Can you work these out from the model? Positions are in its coordinate system, mm. Coordinates: 2 decimals unless noted, no trailing zeros. Write each loop counter-clockwise with the first axis right and the second up, starting at its lowest first coordinate (ties: lowest second). Pieces come first, ordered by that corner, then holes.
```python
from build123d import *

# Parameters (mm, degrees)
SKETCH_1_W      = 200
SKETCH_1_H      = 5
EXTRUDE_1_DEPTH = 3


with BuildPart() as part:
    # 草图1 → 凸台-拉伸1 (new body)
    with BuildSketch(Plane.XY):
        Polygon((0, -80), (0, -100), (100, -100), (100, 0), (80, 0), (80, -3), (40, -3), (40, 0), (0, 0), (0, -40), (3, -40), (3, -80), align=None)
        Polygon((100, -100), (0, -100), (0, -120), (3, -120), (3, -160), (0, -160), (0, -200), (40, -200), (40, -197), (80, -197), (80, -200), (100, -200), align=None)
        Polygon((100, 0), (100, -100), (200, -100), (200, -80), (197, -80), (197, -40), (200, -40), (200, 0), (160, 0), (160, -3), (120, -3), (120, 0), align=None)
        Polygon((200, -100), (100, -100), (100, -200), (120, -200), (120, -197), (160, -197), (160, -200), (200, -200), (200, -160), (197, -160), (197, -120), (200, -120), align=None)
        Polygon((-5, -205), (-5, 5), (0, 5), (0, 0), (0, -200), (0, -205), align=None)
        with Locations((100, 2.5)):
            Rectangle(SKETCH_1_W, SKETCH_1_H)
        Polygon((205, 5), (205, -200), (200, -200), (200, 0), (200, 5), align=None)
        Polygon((0, -200), (200, -200), (205, -200), (205, -205), (0, -205), align=None)
    extrude(amount=EXTRUDE_1_DEPTH)


solid = part.part
```
1. If we section it at B-B, the plane x = 133.5: List the corners of the cut face in (y, z) for me.
2. If I drill on L1, parallel to X at y = -73.5, z = 1.2; L2, parallel to Y at x = 70, z = 0.55, over which ranges is the centre line in solid material (lowest first)?
3. If we section it at C-C, the plane z = 0.65: Count the separate pieces of the cut face and the enclosed holes in it, plus the area to 3 significant figures.
4. If we section it at A-A, the plane y = -75.5: List the corners of the cut face in (x, z) for me, plus the area to 3 significant figures.
Answers:
1. outline: (-205, 0) - (-200, 0) - (-200, 3) - (-205, 3) - close; (-197, 0) - (-3, 0) - (-3, 3) - (-197, 3) - close; (0, 0) - (5, 0) - (5, 3) - (0, 3) - close
2. L1: x = -5 to 0, 3 to 197, 200 to 205
2. L2: y = -205 to -200, -197 to -3, 0 to 5
3. separate pieces: 1
3. enclosed holes: 8
3. area: 43,100 mm2
4. outline: (-5, 0) - (0, 0) - (0, 3) - (-5, 3) - close; (3, 0) - (197, 0) - (197, 3) - (3, 3) - close; (200, 0) - (205, 0) - (205, 3) - (200, 3) - close
4. area: 612 mm2
